Here's how the part is built. I have some questions about the finished solid (model axes, mm). Coordinates: 2 decimals unless noted, no trailing zeros. Use a Markdown table: item, result.
```python
from build123d import *

# Parameters (mm, degrees)
F0_W           = 152.4
F0_H           = 152.4
F1_DEPTH       = 6.35
F3_D           = 6.858
F3_CSINK_D     = 13.716
F3_CSINK_ANGLE = 82


with BuildPart() as f1:
    # F0 (on Front) → F1 (new body)
    with BuildSketch(Plane.XZ):
        with Locations((6.360243, -5.05251)):
            Rectangle(F0_W, F0_H)
    extrude(amount=F1_DEPTH)

    # F3 (through all)
    with Locations(Plane.XZ.offset(6.35)):
        with Locations((-57.139757, 52.09749), (-57.139757, 39.39749), (69.860243, 52.09749), (69.860243, 39.39749), (69.860243, -24.10251), (69.860243, -62.20251), (-57.139757, -62.20251), (-57.139757, -24.10251)):
            CounterSinkHole(F3_D / 2, F3_CSINK_D / 2, counter_sink_angle=F3_CSINK_ANGLE)


solid = f1.part
```
Q1. Will this pin go through, and if not, where does the flat tip stop? P1, Ø11, axis at x = 69.86, z = 52.1, coming from the -Y side.
Check values:
| item | result |
|---|---|
| P1 | y = -4.79 |
Q2. I want a section at A-A, the plane y = -4. Give the number of separate pieces and of enclosed holes in the cut face, then the cut area to 3 significant figures.
Check values:
| item | result |
|---|---|
| separate pieces | 1 |
| enclosed holes | 8 |
| area | 22,600 mm^2 |
Q3. If we mould it in two halves opening along X, with no side actions, what happens to faces 1 (the face through (-69.84, -3, -6)), 2 (the face through (-56.36, -2.597, 35.887)), 3 (the face through (5, -6.35, -4))? For each: pulls with the +X half, pulls with the -X half, needs draft (parallel to the pull), parting line crosses it, or undercut.
Check values:
| item | result |
|---|---|
| face 1 | pulls with the -X half |
| face 2 | undercut |
| face 3 | needs draft |
Q4. Please list where these lines run through material, in increasing order: L1, parallel to X at y = -5, z = -20.5; L2, parallel to X at y = -4.75, z = -22.5; L3, parallel to Z at x = -63, y = -6. Write a range as from..to.
Check values:
| item | result |
|---|---|
| L1 | -69.84..-61.54, -52.74..65.46, 74.26..82.56 |
| L2 | -69.84..-62.37, -51.91..64.63, 75.09..82.56 |
| L3 | -81.25..-65.14, -59.27..-27.04, -21.17..36.46, 42.33..49.16, 55.03..71.15 |
